Verification items for the finished model (mm, model axes). A direction names the side the tool comes from. Round coordinates to 2 decimals unless told otherwise and drop trailing zeros. Write each loop counter-clockwise with the first axis right and the second up, starting at its lowest first coordinate (ties: lowest second). Pieces come first, ordered by that corner, then holes. Notation, with made-up numbers: M -34.75,24.25 L -0.75,24.25 A22 ccw -0.75,36.25 Z; hole C -10,83.5 d11. An arc over 180 degrees is marked long. Answer in a Markdown table with one row per item. Add a question column.
1. Draft check along X on faces 1 (the conical face through (0.42, -0.13, -1.51)), 2 (the flat face through (-7.541, -3, 0)), 3 (the flat face through (-3, 7.541, 0)), 4 (the cylindrical face through (-2.435, -0.767, -5.126)). Enter one of: pulls with the +X half, pulls with the -X half, needs draft (parallel to the pull), parting line crosses it, or undercut.
2. Material ranges on probe 1 along Y at (x, z) = (0, -5.2), recorded low to high.
3. Sectioned sample at A-A on z = -5. Record the cut outline in (x, y).
4. Set-up check for faces 5 (the flat face through (-3, 0, -7.541)), 6 (the cylindrical face through (-5.126, 2.435, 0.767)), 7 (the cylindrical face through (2.435, 5.126, 0.767)): record each of +Z, -Z, +X, -X, +Y, -Y from which the full face is reachable in a straight line by a thin tool's end or side.
```python
from build123d import *

# Parameters (mm, degrees)
F0_W     = 15.08125
F0_H     = 15.08125
F1_DEPTH = 7.540625
F5_D     = 5.1054
F5_DEPTH = 4.7625
F5_TIP   = 1.5338169022
F6_D     = 5.1054
F6_DEPTH = 4.7625
F6_TIP   = 1.5338169022
F7_D     = 5.1054
F7_DEPTH = 4.7625
F7_TIP   = 1.5338169022


with BuildPart() as f1:
    # F0 (on Top) → F1 (new body, symmetric)
    with BuildSketch(Plane.XY):
        Rectangle(F0_W, F0_H)
    extrude(amount=F1_DEPTH, both=True)

    # F5
    with Locations(Plane(origin=(0, 0, -7.540625), x_dir=(1, 0, 0), z_dir=(0, 0, -1))):
        with Locations((0, 0)):
            Hole(F5_D / 2, depth=F5_DEPTH)
            with Locations((0, 0, -(F5_DEPTH + F5_TIP / 2))):  # 118° drill point
                Cone(0, F5_D / 2, F5_TIP, mode=Mode.SUBTRACT)

    # F6
    with Locations(Plane(origin=(0, 7.540625, 0), x_dir=(-1, 0, 0), z_dir=(0, 1, 0))):
        with Locations((0, 0)):
            Hole(F6_D / 2, depth=F6_DEPTH)
            with Locations((0, 0, -(F6_DEPTH + F6_TIP / 2))):  # 118° drill point
                Cone(0, F6_D / 2, F6_TIP, mode=Mode.SUBTRACT)

    # F7
    with Locations(Plane(origin=(-7.540625, 0, 0), x_dir=(0, -1, 0), z_dir=(-1, 0, 0))):
        with Locations((0, 0)):
            Hole(F7_D / 2, depth=F7_DEPTH)
            with Locations((0, 0, -(F7_DEPTH + F7_TIP / 2))):  # 118° drill point
                Cone(0, F7_D / 2, F7_TIP, mode=Mode.SUBTRACT)


solid = f1.part
```
Geometry check:
| question | item | result |
|---|---|---|
| 1 | face 1 | undercut |
| 1 | face 2 | pulls with the -X half |
| 1 | face 3 | needs draft |
| 1 | face 4 | undercut |
| 2 | probe 1 | y = -7.54 to -2.55, 2.55 to 7.54 |
| 3 | outline | M -7.54,-7.54 L 7.54,-7.54 L 7.54,7.54 L -7.54,7.54 Z; hole C 0,0 d5.11 |
| 4 | face 5 | -Z, +X, -X, +Y, -Y |
| 4 | face 6 | -X |
| 4 | face 7 | +Y |
